Can you work these out from the drawing? Everything is in mm from the part's minimum corner. A direction names the side the tool comes from. Coordinates: 2 decimals unless noted, no trailing zeros. Loops run counter-clockwise (first coordinate to the right, second up) from the corner with the lowest first, then second, coordinate; pieces in that order, holes last.
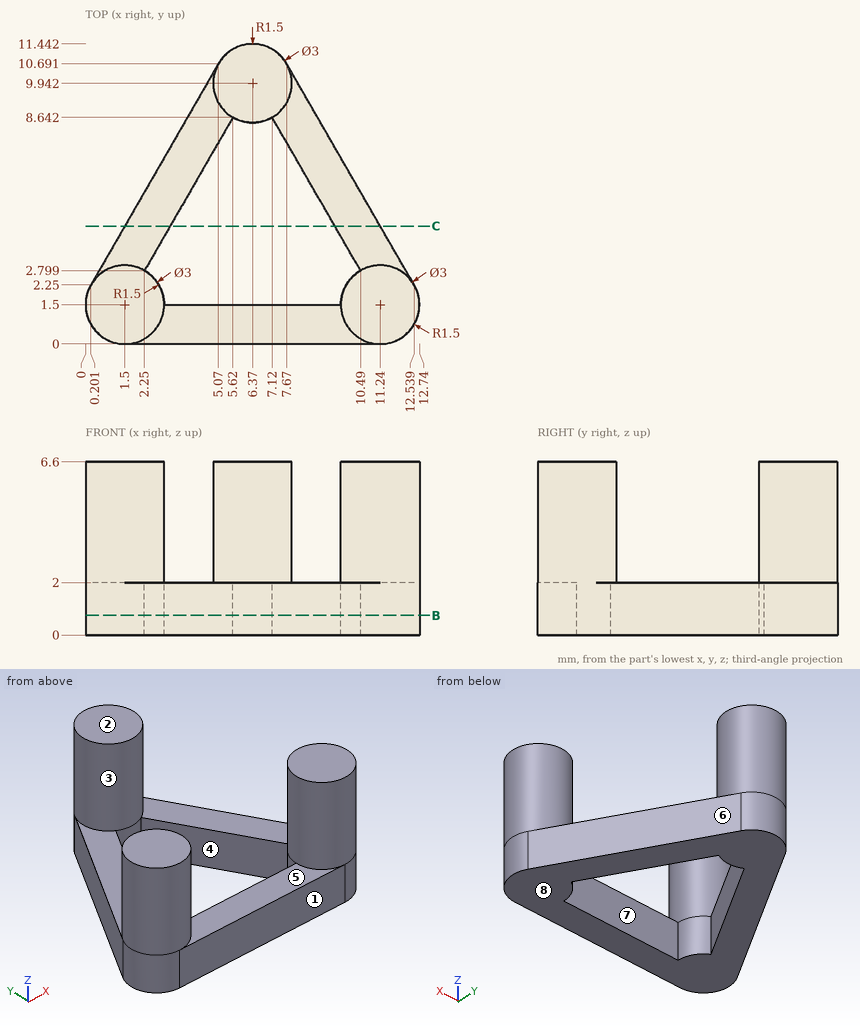
Item 1: I'm going to push flat-ended pins straight in: P1, Ø2, axis at y = 8.5, z = 5, coming from the -X side; P2, Ø1, axis at x = 7, z = 4.5, coming from the +Y side; P3, Ø6, axis at x = 2.5, y = 4, coming from the -Z side; P4, Ø3, axis at x = 5.5, y = 6.5, coming from the +Z side. Where does each tip first touch, or does it pass through?
Results are:
P1: stops at x = 4.94
P2: stops at y = 11.44
P3: stops at z = 0
P4: stops at z = 2
Item 2: Suppose I cut it at B-B, the plane z = 0.75. Please give me the cut outline in (x, y).
Results are:
outline: (0.2, 2.25) arc R1.5 ccw to (1.5, 0) - (11.24, 0) arc R1.5 ccw to (12.54, 2.25) - (7.67, 10.69) arc R1.5 ccw to (5.07, 10.69) - close; hole (2.25, 2.8) arc R1.5 cw to (3, 1.5) - (9.74, 1.5) arc R1.5 cw to (10.49, 2.8) - (7.12, 8.64) arc R1.5 cw to (5.62, 8.64) - close
Item 3: Suppose I cut it at C-C, the plane y = 4.5. Please give me the cut outline in (x, z).
Results are:
outline: (1.5, 0) - (3.23, 0) - (3.23, 2) - (1.5, 2) - close; (9.51, 0) - (11.24, 0) - (11.24, 2) - (9.51, 2) - close
Item 4: On a 3-axis mill with a long thin cutter (end or side, diameter ignored), from which of +Z, -Z, +X, -X, +Y, -Y can I reach the whole of each face in a straight line? I mean the marked faces 1, 2, 3, 4 and 5. Say none if no direction works.
Results are:
face 1: +Z, -Z, +X, -X, -Y
face 2: +Z, +X, -X, +Y, -Y
face 3: +Z
face 4: +Z, -Z
face 5: +Z, -Y
Item 5: We'd pull the mould along X, two halves only. Please class the marked faces 6, 7 and 8: +X half, -X half, draft (parallel to the pull), parting line (faces both ways), or undercut.
Results are:
face 6: +X half
face 7: undercut
face 8: draft
Item 6: I need wall thicknesses on line 1 along X through (y, z) = (2.75, 3.5); line 2 along X through (y, z) = (4.5, 0.75); line 3 along Y through (x, z) = (4, 1.5) (1 decimal). Which ranges of each line are inside material? Lowest first, please.
Results are:
line 1: x = 0.67 to 2.33, 10.41 to 12.07
line 2: x = 1.5 to 3.23, 9.51 to 11.24
line 3: y = 0 to 1.5, 5.8 to 8.8
